from build123d import *

# Parameters (mm, degrees)
SKETCH1_W                                       = 95.25
SKETCH1_H                                       = 231.8385
EXTRUDE1_DEPTH                                  = 9.525
CSK_FOR_M8_FLAT_HEAD_MACHINE_SCREW1_AT_2_COUNT  = 2
CSK_FOR_M8_FLAT_HEAD_MACHINE_SCREW1_AT_2_PITCH  = 25.4
CSK_FOR_M8_FLAT_HEAD_MACHINE_SCREW2_D           = 9
CSK_FOR_M8_FLAT_HEAD_MACHINE_SCREW2_CSINK_D     = 17.3
CSK_FOR_M8_FLAT_HEAD_MACHINE_SCREW2_CSINK_ANGLE = 90
CUT_EXTRUDE1_REACH                              = 11.525
BOSS_EXTRUDE1_DEPTH                             = 9.525
FILLET1_R                                       = 9.525
FILLET2_R                                       = 19.05


with BuildPart() as part:
    # Sketch1 → Extrude1 (new body)
    with BuildSketch(Plane.XY):
        Rectangle(SKETCH1_W, SKETCH1_H)
    extrude(amount=EXTRUDE1_DEPTH)

    # Sketch2 → CSK for M8 Flat Head Machine Screw1 (revolve, cut)
    with BuildSketch(Plane(origin=(31.75, -50.15865, 9.525), x_dir=(0, -1, 0), z_dir=(1, 0, 0))):
        Polygon((0, 0), (0, 9.525), (4.5, 9.525), (4.5, 8.1124), (8.65, 3.9624), (8.65, 0), align=None)
    csk_for_m8_flat_head_machine_screw1 = revolve(axis=Axis((31.75, -50.15865, 15.875), (0, 0, -1)), mode=Mode.SUBTRACT)

    # CSK for M8 Flat Head Machine Screw1 at 2: CSK for M8 Flat Head Machine Screw1 ×2
    with Locations(*[(0, i * CSK_FOR_M8_FLAT_HEAD_MACHINE_SCREW1_AT_2_PITCH, 0) for i in range(1, CSK_FOR_M8_FLAT_HEAD_MACHINE_SCREW1_AT_2_COUNT)]):
        add(csk_for_m8_flat_head_machine_screw1, mode=Mode.SUBTRACT)

    # CSK for M8 Flat Head Machine Screw2 (through all)
    with Locations(Plane.XY.offset(9.525)):
        with Locations((-34.925, 103.21925), (-34.925, -103.21925)):
            CounterSinkHole(CSK_FOR_M8_FLAT_HEAD_MACHINE_SCREW2_D / 2, CSK_FOR_M8_FLAT_HEAD_MACHINE_SCREW2_CSINK_D / 2, counter_sink_angle=CSK_FOR_M8_FLAT_HEAD_MACHINE_SCREW2_CSINK_ANGLE)

    # Sketch11 → Cut-Extrude1 (cut, up to next)
    with BuildSketch(Plane.XY.offset(9.525), mode=Mode.PRIVATE) as cut_extrude1_sk1:
        Polygon((-47.625, 115.91925), (47.625, 113.425040971), (47.625, 115.91925), align=None)
    cut_extrude1_tool1 = extrude(cut_extrude1_sk1.sketch, amount=-CUT_EXTRUDE1_REACH, mode=Mode.PRIVATE) & part.part
    add(cut_extrude1_tool1.solids().sort_by_distance((15.875, 115.087847, 9.525))[0], mode=Mode.SUBTRACT)
    # Sketch11 → Cut-Extrude1 (cut, up to next)
    with BuildSketch(Plane.XY.offset(9.525), mode=Mode.PRIVATE) as cut_extrude1_sk2:
        Polygon((-47.625, -115.91925), (47.625, -115.91925), (47.625, -113.425040971), align=None)
    cut_extrude1_tool2 = extrude(cut_extrude1_sk2.sketch, amount=-CUT_EXTRUDE1_REACH, mode=Mode.PRIVATE) & part.part
    add(cut_extrude1_tool2.solids().sort_by_distance((15.875, -115.087847, 9.525))[0], mode=Mode.SUBTRACT)

    # Sketch12 → Boss-Extrude1 (add)
    with BuildSketch(Plane.XY.offset(9.525)):
        Polygon((47.625, 113.425040971), (193.675, 109.600587125), (193.675, 71.500587125), (47.625, 71.500587125), align=None)
        Polygon((47.625, -71.500587125), (193.675, -71.500587125), (193.675, -109.600587125), (47.625, -113.425040971), align=None)
    extrude(amount=-BOSS_EXTRUDE1_DEPTH)

    # Fillet1
    fillet1_edges = [part.edges().sort_by_distance(p)[0] for p in [
        (193.675, 109.600587125, 4.7625),
        (193.675, 71.500587125, 4.7625),
        (193.675, -71.500587125, 4.7625),
        (193.675, -109.600587125, 4.7625),
    ]]
    fillet(fillet1_edges, radius=FILLET1_R)

    # Fillet2
    fillet2_edges = [part.edges().sort_by_distance(p)[0] for p in [
        (47.625, 71.500587125, 4.7625),
        (47.625, -71.500587125, 4.7625),
    ]]
    fillet(fillet2_edges, radius=FILLET2_R)


solid = part.part
Build history of the part. All positions in model axes, mm. A direction names the side the tool comes from. Coordinates: 2 decimals unless noted, no trailing zeros. Write each loop counter-clockwise with the first axis right and the second up, starting at its lowest first coordinate (ties: lowest second). Pieces come first, ordered by that corner, then holes. Notation, with made-up numbers: (40.5, 10) -> (82.5, 10) arc R14 cw to (82.5, 18) -> close; hole circle Ø10 at (-28.75, 85.25). An arc over 180 degrees is marked (long way). Use CSV: the item, a comma, the result in double quotes. Start each with the question number.
Q1. Cut at A-A, the plane x = 107.5. List the corners of the cut face in (y, z) (3 decimals).
Q2. 3-axis set-ups, long thin cutter, end or side, ignore diameter. For faces 1 (the flat face through (-47.625, -2, 5)), 2 (the cylindrical face through (25.904, -43.783, 7.572)), 3 (the flat face through (47.625, -1, 5)): which of +Z, -Z, +X, -X, +Y, -Y reach the whole face in a straight line?
Q3. Flat gauge pins, fed straight in: pin 1 Ø1 at (x, z) = (150, 4) entering from -Y; pin 2 Ø4 at (x, z) = (156, 8.5) entering from -Y; pin 3 Ø3 at (x, z) = (137, 2.5) entering from +Y. Where does each tip first touch, or does it go through?
Q4. Cut at B-B, the plane x = 31.75. List the corners of the cut face in (y, z) (3 decimals).
Q5. Cut at C-C, the plane y = -68.5. List the corners of the cut face in (x, z) (1 decimal), then the cut area to 3 significant figures.
Q6. Cut at D-D, the plane y = 65. List the corners of the cut face in (x, z) (3 decimals).
Q7. Drill centre lines: probe 1 along Y at (x, z) = (31.75, 6.45); probe 2 along Y at (x, z) = (31.75, 0.6); probe 3 along Y at (x, z) = (142, 7). Where is each one in solid material? Low to high.
Q8. Pull direction Y, two halves, no side cores. Call faces 4 (the cylindrical face through (190.9, 107.04, 4.7)), 5 (the conical face through (33.573, -54.555, 1.672)), 6 (the cylindrical face through (191.044, -106.894, 4.696)): released by +Y, released by -Y, zero draft, split by the parting line, or undercut.
Checked values:
1,outline,"(-111.857, 0) -> (-71.501, 0) -> (-71.501, 9.525) -> (-111.857, 9.525) -> close; (71.501, 0) -> (111.857, 0) -> (111.857, 9.525) -> (71.501, 9.525) -> close"
2,face 1,"+Z, -Z, -X, +Y, -Y"
2,face 2,"+Z"
2,face 3,"+Z, -Z, +X"
3,pin 1,"stops at y = -110.76"
3,pin 2,"stops at y = -110.64"
3,pin 3,"stops at y = 111.12"
4,outline,"(-113.841, 0) -> (-54.659, 0) -> (-54.659, 1.413) -> (-58.809, 5.563) -> (-58.809, 9.525) -> (-113.841, 9.525) -> close; (-45.659, 0) -> (-29.259, 0) -> (-29.259, 1.413) -> (-33.409, 5.563) -> (-33.409, 9.525) -> (-41.509, 9.525) -> (-41.509, 5.563) -> (-45.659, 1.413) -> close; (-20.259, 0) -> (113.841, 0) -> (113.841, 9.525) -> (-16.109, 9.525) -> (-16.109, 5.563) -> (-20.259, 1.413) -> close"
5,outline,"(-47.6, 0) -> (56.4, 0) -> (56.4, 9.5) -> (-47.6, 9.5) -> close"
5,area,"991 mm²"
6,outline,"(-47.625, 0) -> (52.343, 0) -> (52.343, 9.525) -> (-47.625, 9.525) -> close"
7,probe 1,"y = -113.84 to -58.81, -41.51 to -33.41, -16.11 to 113.84"
7,probe 2,"y = -113.84 to -54.66, -45.66 to -29.26, -20.26 to 113.84"
7,probe 3,"y = -110.95 to -71.5, 71.5 to 110.95"
8,face 4,"released by +Y"
8,face 5,"undercut"
8,face 6,"released by -Y"
